from build123d import *

# Parameters (mm, degrees)
F0_W     = 39.6875
F0_H     = 39.6875
F0_R     = 12.8778
F0_R_2   = 11.2268
F1_DEPTH = 7.9375
F2_DEPTH = 2.032
F3_D     = 5.1054


with BuildPart() as f1:
    # F0 (on Top) → F1 (new body)
    with BuildSketch(Plane.XY):
        Rectangle(F0_W, F0_H)
        Circle(F0_R, mode=Mode.SUBTRACT)
        Circle(F0_R)
        Circle(F0_R_2, mode=Mode.SUBTRACT)
        Circle(F0_R_2)
    extrude(amount=-F1_DEPTH)

    # F0 (on Top) → F2 (cut)
    with BuildSketch(Plane.XY):
        Circle(F0_R)
        Circle(F0_R_2, mode=Mode.SUBTRACT)
    extrude(amount=-F2_DEPTH, mode=Mode.SUBTRACT)

    # F3 (through all)
    with Locations(Plane.XY):
        with Locations((-15.08125, 15.08125), (15.08125, 15.08125), (15.08125, -15.08125), (-15.08125, -15.08125)):
            Hole(F3_D / 2)


solid = f1.part
Could you check a few things on this model? Use its own coordinates, in mm. A direction names the side the tool comes from. Coordinates: 2 decimals unless noted, no trailing zeros. Write each loop counter-clockwise with the first axis right and the second up, starting at its lowest first coordinate (ties: lowest second). Pieces come first, ordered by that corner, then holes. Notation, with made-up numbers: M 84.5,-10.5 L 110.5,-10.5 A18 cw 110.5,12.5 Z; hole C 31.5,46 d7. An arc over 180 degrees is marked long. One line per question, with ' | ' between items.
1) For pin 1 Ø4 at (x, y) = (-15.08, -15.08) entering from +Z (3 decimals), with a flat end and sliding along its axis, tell me the tip position at first contact or that it passes through.
Checks:
pin 1: through
2) Imagine slicing it at A-A, the plane y = 16. Write out the boundary of the cut face in (x, z).
Checks:
outline: M -19.84,-7.94 L -17.46,-7.94 L -17.46,0 L -19.84,0 Z; M -12.7,-7.94 L 12.7,-7.94 L 12.7,0 L -12.7,0 Z; M 17.46,-7.94 L 19.84,-7.94 L 19.84,0 L 17.46,0 Z
3) Imagine slicing it at C-C, the plane y = 0. Write out the boundary of the cut face in (x, z).
Checks:
outline: M -19.84,-7.94 L 19.84,-7.94 L 19.84,0 L 12.88,0 L 12.88,-2.03 L 11.23,-2.03 L 11.23,0 L -11.23,0 L -11.23,-2.03 L -12.88,-2.03 L -12.88,0 L -19.84,0 Z
4) I need wall thicknesses on probe 1 along Y at (x, z) = (-2, -1.25); probe 2 along X at (y, z) = (-14.5, -1.5); probe 3 along X at (y, z) = (-9.5, -1). Which ranges of each line are inside material? Lowest first, please. Write a range as [from, to].
Checks:
probe 1: [-19.84, -12.72], [-11.05, 11.05], [12.72, 19.84] | probe 2: [-19.84, -17.57], [-12.6, 12.6], [17.57, 19.84] | probe 3: [-19.84, -8.69], [-5.98, 5.98], [8.69, 19.84]
5) If we mould it in two halves opening along Y, with no side actions, what happens to faces 3 (the face through (19.844, 0, -4)), 4 (the face through (-4, 11, -2.032)), 5 (the face through (0, 19.844, -4))? For each: released by +Y, released by -Y, zero draft, split by the parting line, or undercut.
Checks:
face 3: zero draft | face 4: undercut | face 5: released by +Y
6) Imagine slicing it at B-B, the plane z = -1.25. Write out the boundary of the cut face in (x, y), and give its area (3 significant figures).
Checks:
outline: M -19.84,-19.84 L 19.84,-19.84 L 19.84,19.84 L -19.84,19.84 Z; C 0,0 d22.45; hole C -15.08,-15.08 d5.11; hole C -15.08,15.08 d5.11; hole C 0,0 d25.76; hole C 15.08,-15.08 d5.11; hole C 15.08,15.08 d5.11 | area: 1,370 mm²
7) For faces 1 (the face through (12.723, -16.059, -4.024)), 2 (the face through (12.283, 3.868, -1.002)), which set-ups out of +Z, -Z, +X, -X, +Y, -Y let a thin tool reach every point of the face, with its end or its side?
Checks:
face 1: +Z, -Z | face 2: +Z
